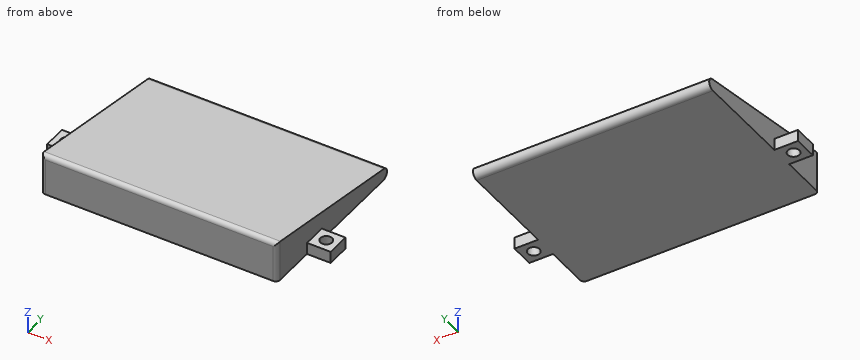
from build123d import *

# Parameters (mm, degrees)
F1_DEPTH = 127
F2_W     = 12.7
F2_H     = 6.35
F3_DEPTH = 12.7
F4_W     = 12.7
F4_H     = 6.35
F5_DEPTH = 12.7
F6_R     = 3.175
F7_DEPTH = 6.351
F8_R     = 3.175
F9_DEPTH = 6.351
F10_R    = 3.175
F11_R    = 2.2225


with BuildPart() as f1:
    # F0 (on Right) → F1 (new body)
    with BuildSketch(Plane.YZ):
        Polygon((-127, 0), (0, 0), (-127, 22.393527), align=None)
    extrude(amount=F1_DEPTH)

    # F2 (on face) → F3 (join)
    with BuildSketch(Plane.YZ.offset(127)):
        with Locations((-95.25, 3.175)):
            Rectangle(F2_W, F2_H)
    extrude(amount=F3_DEPTH)

    # F4 (on face) → F5 (join)
    with BuildSketch(Plane(origin=(0, 0, 0), x_dir=(0, -1, 0), z_dir=(-1, 0, 0))):
        with Locations((95.25, 3.175)):
            Rectangle(F4_W, F4_H)
    extrude(amount=F5_DEPTH)

    # F6 (on face) → F7 (cut, through all)
    with BuildSketch(Plane.XY.offset(6.35)):
        with Locations((-6.35, -95.25)):
            Circle(F6_R)
    extrude(amount=-F7_DEPTH, mode=Mode.SUBTRACT)

    # F8 (on face) → F9 (cut, through all)
    with BuildSketch(Plane.XY.offset(6.35)):
        with Locations((133.35, -95.25)):
            Circle(F8_R)
    extrude(amount=-F9_DEPTH, mode=Mode.SUBTRACT)

    # F10
    f10_edges = [f1.edges().sort_by_distance(p)[0] for p in [
        (63.5, 0, 0),
    ]]
    fillet(f10_edges, radius=F10_R)

    # F11
    f11_edges = [f1.edges().sort_by_distance(p)[0] for p in [
        (63.5, -127, 22.393527),
        (127, -127, 11.196763),
        (0, -127, 11.196763),
    ]]
    fillet(f11_edges, radius=F11_R)


solid = f1.part
For this review, take the finished solid that the model builds, in its own axes (mm). Round coordinates to 2 decimals unless told otherwise and drop trailing zeros. Order: outer loops, then holes, each group sorted by start corner. A loop starts at its lowest first (then second) coordinate and runs counter-clockwise, first axis right, second up. Notation, with made-up numbers: M -31,74 L 22,74 A26 ccw 22,109 Z; hole C 78,32.25 d4. An arc over 180 degrees is marked long. Write each question's results on one line, items separated by ' | '. Start each with the question number.
1. Clearance check with flat-ended pins moving along their axes: pin 1 Ø2 at (x, z) = (105, 6.5) entering from +Y; pin 2 Ø8 at (y, z) = (-95, 16.5) entering from +X; pin 3 Ø1.9 at (x, z) = (131.5, 4.5) entering from +Y; pin 4 Ø4 at (x, y) = (-6.35, -95.25) entering from +Z. State where each tip first meets the part, or that it passes through.
2. Add section C-C (z = 2). State how many separate pieces and enclosed holes the cut face has, then the cut area to 3 significant figures.
3. Add section A-A (x = 133.35). State the section outline as (y, z) points (3 decimals).
4. To check wall thickness, follow L1, parallel to Y at x = -6.35, z = 2 (3 decimals); L2, parallel to X at y = -113, z = 10.25; L3, parallel to Y at x = 9, z = 2.5. State the ranges of each line that lie inside material, in increasing order. Write a range as [from, to].
5. Add section B-B (y = -95.25). State the section outline as (x, z) points (3 decimals), then the cut area to 3 significant figures.
Output values:
1) pin 1: y = -34.13 | pin 2: x = 127 | pin 3: y = -88.9 | pin 4: through
2) separate pieces: 1 | enclosed holes: 2 | area: 12,200 mm^2
3) outline: M -101.6,0 L -98.425,0 L -98.425,6.35 L -101.6,6.35 Z; M -92.075,0 L -88.9,0 L -88.9,6.35 L -92.075,6.35 Z
4) L1: [-101.6, -98.425], [-92.075, -88.9] | L2: [0, 127] | L3: [-127, -33.19]
5) outline: M -12.7,0 L -9.525,0 L -9.525,6.35 L -12.7,6.35 Z; M -3.175,0 L 130.175,0 L 130.175,6.35 L 127,6.35 L 127,16.795 L 0,16.795 L 0,6.35 L -3.175,6.35 Z; M 136.525,0 L 139.7,0 L 139.7,6.35 L 136.525,6.35 Z | area: 2,210 mm^2
